Source: three-view drawing plus pictorial views. Frame: mm from the lowest corner of the part. A direction names the side the tool comes from. Round coordinates to 2 decimals unless told otherwise and drop trailing zeros. Loops run counter-clockwise (first coordinate to the right, second up) from the corner with the lowest first, then second, coordinate; pieces in that order, holes last. Notation, with made-up numbers: M 25.5,21 L 29.5,21 A16 ccw 29.5,36 Z; hole C -19,71.25 d6. An arc over 180 degrees is marked long. Write each question's results on one line, items separated by ' | '.
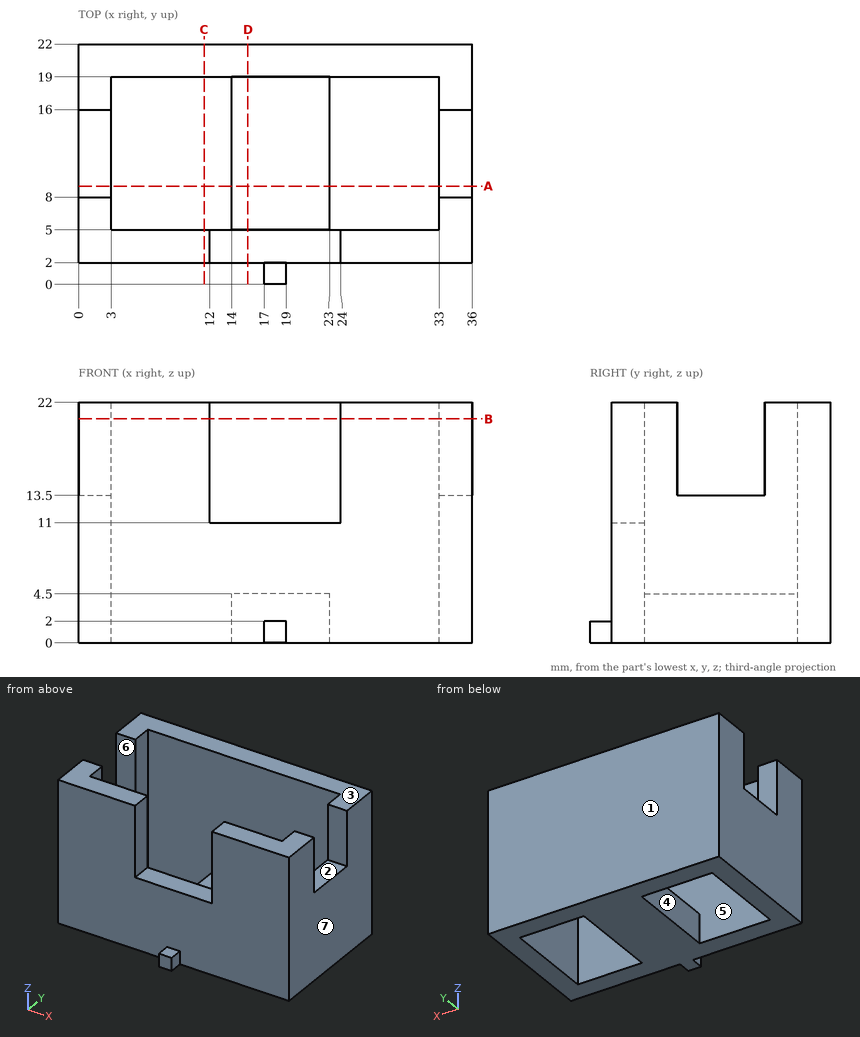
1. Section A-A (y = 9). Output: boundary loops of the cut face in (x, z), then the cut area to 4 significant figures.
Answer key:
outline: M 0,0 L 3,0 L 3,13.5 L 0,13.5 Z; M 14,0 L 23,0 L 23,4.5 L 14,4.5 Z; M 33,0 L 36,0 L 36,13.5 L 33,13.5 Z | area: 121.5 mm²
2. Draft query along Y for the marked faces 1, 2 and 3. Return one class per face: pulls with the +Y half, pulls with the -Y half, needs draft (parallel to the pull), parting line crosses it, or undercut.
Answer key:
face 1: pulls with the +Y half | face 2: undercut | face 3: needs draft
3. Section C-C (x = 11.5). Output: boundary loops of the cut face in (y, z).
Answer key:
outline: M 2,0 L 5,0 L 5,22 L 2,22 Z; M 19,0 L 22,0 L 22,22 L 19,22 Z
4. Pin query (flat end, axial travel): P1, Ø0.6, axis at x = 18, y = 1, coming from the +Z side; P2, Ø2, axis at x = 25, z = 15, coming from the -Y side; P3, Ø10, axis at y = 6, z = 16, coming from the -X side; P4, Ø1.5, axis at x = 18, y = 4, coming from the +Z side. Return the tip coordinate at first contact, or that it passes through.
Answer key:
P1: stops at z = 2 | P2: stops at y = 2 | P3: stops at x = 0 | P4: stops at z = 11
5. Section B-B (z = 20.5). Output: boundary loops of the cut face in (x, y), then the cut area to 3 significant figures.
Answer key:
outline: M 0,2 L 12,2 L 12,5 L 3,5 L 3,8 L 0,8 Z; M 0,16 L 3,16 L 3,19 L 33,19 L 33,16 L 36,16 L 36,22 L 0,22 Z; M 24,2 L 36,2 L 36,8 L 33,8 L 33,5 L 24,5 Z | area: 216 mm²
6. Access query for the marked faces 4, 5, 6 and 7. Directions: +Z, -Z, +X, -X, +Y, -Y. A direction counts if a zero-diameter tool reaches every point of the face in a straight line with its end or side. Return the directions, or none.
Answer key:
face 4: +Z, -Z | face 5: +Z | face 6: +Z, +X, -X | face 7: +Z, -Z, +X, +Y, -Y
7. Ray query, probe 1 along X at (y, z) = (6, 2.25); probe 2 along Y at (x, z) = (5.5, 7.5); probe 3 along X at (y, z) = (5.75, 17.75). Return the intervals inside material, ascending.
Answer key:
probe 1: x = 0 to 3, 14 to 23, 33 to 36 | probe 2: y = 2 to 5, 19 to 22 | probe 3: x = 0 to 3, 33 to 36
8. Section D-D (x = 15.5). Output: boundary loops of the cut face in (y, z).
Answer key:
outline: M 2,0 L 22,0 L 22,22 L 19,22 L 19,4.5 L 5,4.5 L 5,11 L 2,11 Z
